The figure shows three views and two pictorial views of one solid part (mm, origin at its lowest corner). Answer the questions. A direction names the side the tool comes from. Give positions to 0.01 mm unless a question says otherwise; leave off trailing zeros. Order: outer loops, then holes, each group sorted by start corner. A loop starts at its lowest first (then second) coordinate and runs counter-clockwise, first axis right, second up. Notation, with made-up numbers: M 50,46 L 68,46 A19 ccw 68,64 Z; hole C 81,-14.75 d5. An arc over 180 degrees is marked long. One line per item, written item: value. Start each with the question number.
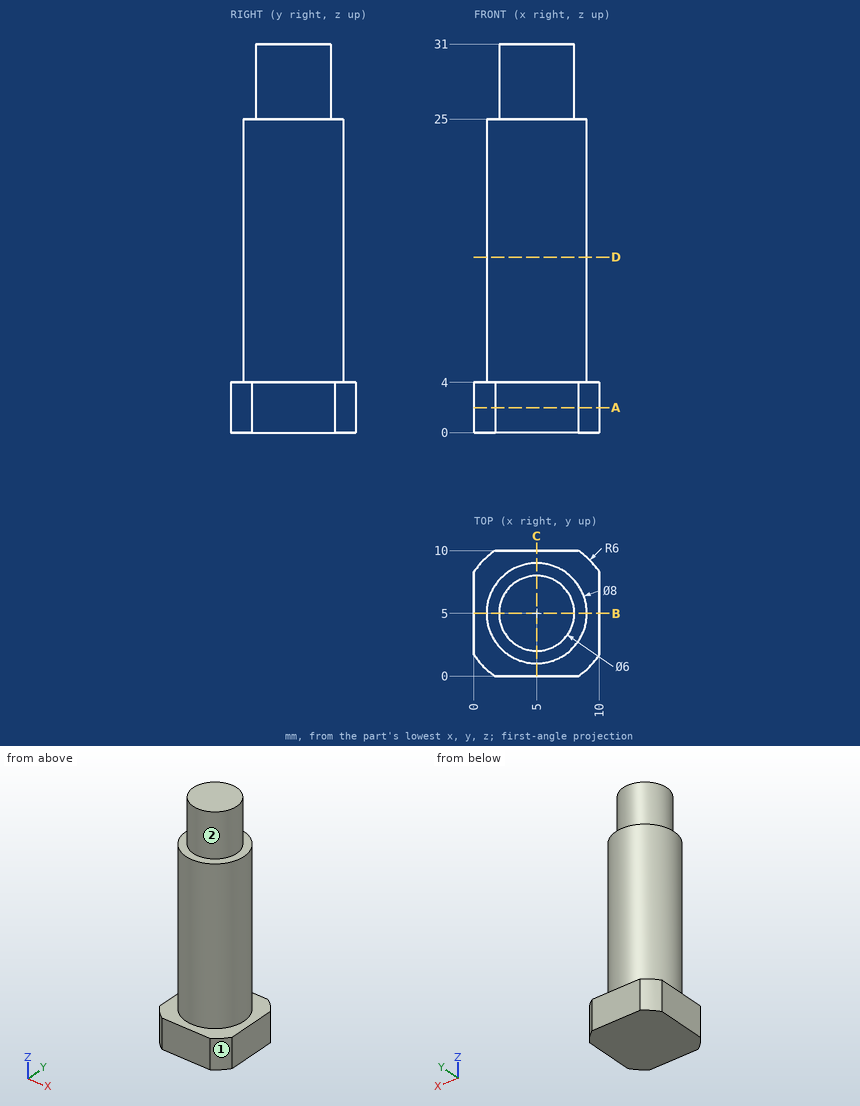
Q1. Consider probe 1 along Z at (x, y) = (8.5, 8.5); probe 2 along Z at (x, y) = (8.5, 5.75); probe 3 along X at (y, z) = (5.75, 19). Determine where each line is inside the solid, lowest interval first.
Q2. Find section B-B, the plane y = 5. Give the vertices of the cut face in (x, z).
Q3. A tool of negligible diameter and unlimited length cuts with its end or side. For the marked faces 1 and 2, from which of +Z, -Z, +X, -X, +Y, -Y can it reach the whole face along a straight path? Write none if from no direction.
Q4. Each of these flat-tipped pins is pushed along its axis until it touches: pin 1 (3 mm diameter, centred on x = 1, y = 8.5, fed in from -Z); pin 2 (3 mm diameter, centred on x = 6, z = 27, fed in from -Y); pin 3 (6 mm diameter, centred on y = 1, z = 12, fed in from +X). Where does it stop, or does it pass through?
Q5. Find section A-A, the plane z = 2. Give the vertices of the cut face in (x, y).
Q6. Find section D-D, the plane z = 14. Give the vertices of the cut face in (x, y).
Evaluation:
1. probe 1: 0 to 4
1. probe 2: 0 to 25
1. probe 3: 1.07 to 8.93
2. outline: M 0,0 L 10,0 L 10,4 L 9,4 L 9,25 L 8,25 L 8,31 L 2,31 L 2,25 L 1,25 L 1,4 L 0,4 Z
3. face 1: +Z, -Z, +X, -Y
3. face 2: +Z
4. pin 1: z = 0
4. pin 2: y = 2
4. pin 3: x = 8.87
5. outline: M 0,1.68 A6 ccw 1.68,0 L 8.32,0 A6 ccw 10,1.68 L 10,8.32 A6 ccw 8.32,10 L 1.68,10 A6 ccw 0,8.32 Z
6. outline: C 5,5 d8
